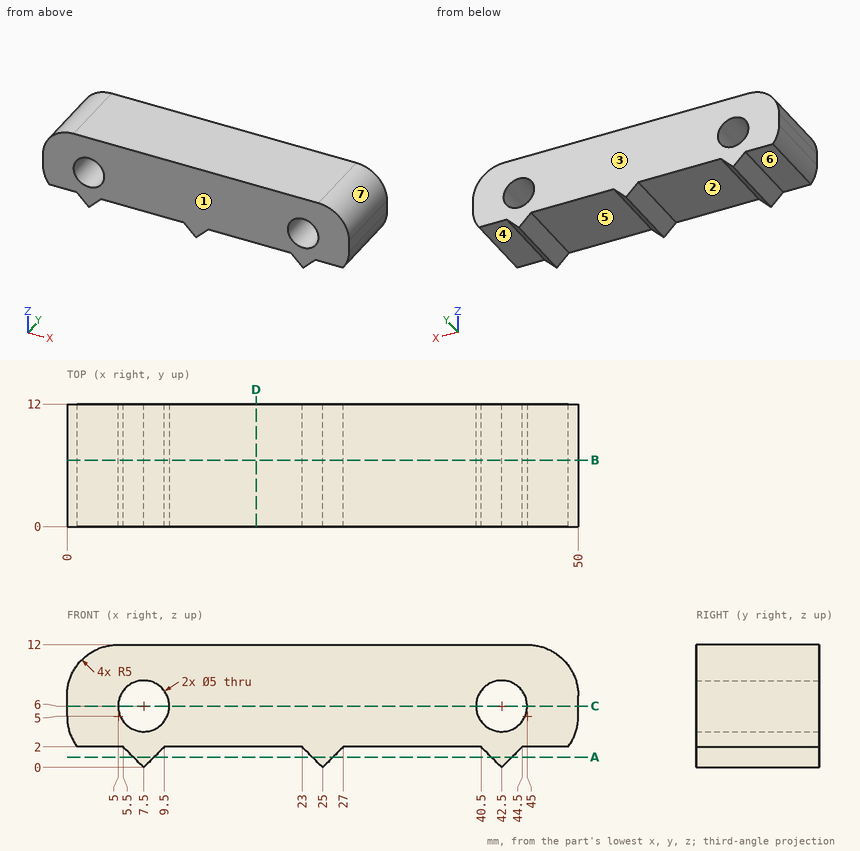
Input: dimensioned drawing with shaded views. Units: mm. Origin: part minimum x, y, z. A direction names the side the tool comes from. Give positions to 0.01 mm unless a question says otherwise; leave off trailing zeros. Write each loop counter-clockwise with the first axis right and the second up, starting at its lowest first coordinate (ties: lowest second). Pieces come first, ordered by that corner, then holes. Notation, with made-up numbers: (-1.5, 3.25) -> (29.5, 3.25) arc R28 ccw to (29.5, 39.25) -> close; hole circle Ø1 at (62, -13). An arc over 180 degrees is marked (long way). Answer as a JSON object with one key per item and string values.
1. Mould query, pull axis Y, two halves, no side actions, for the marked faces 1, 2 and 3. Classes: pulls with the +Y half, pulls with the -Y half, needs draft (parallel to the pull), parting line crosses it, or undercut.
Ans:
{"face 1": "pulls with the -Y half", "face 2": "needs draft", "face 3": "pulls with the +Y half"}
2. Cut plane A-A on z = 1. Output: boundary loops of the cut face in (x, y), and give its area (3 significant figures).
Ans:
{"outline": "(6.5, 0) -> (8.5, 0) -> (8.5, 12) -> (6.5, 12) -> close; (24, 0) -> (26, 0) -> (26, 12) -> (24, 12) -> close; (41.5, 0) -> (43.5, 0) -> (43.5, 12) -> (41.5, 12) -> close", "area": "72.0 mm^2"}
3. Access query for the marked faces 4, 5, 6 and 7. Directions: +Z, -Z, +X, -X, +Y, -Y. A direction counts if a zero-diameter tool reaches every point of the face in a straight line with its end or side. Return the directions, or none.
Ans:
{"face 4": "-Z, +X, +Y, -Y", "face 5": "-Z, +Y, -Y", "face 6": "-Z, -X, +Y, -Y", "face 7": "+Z, +X, +Y, -Y"}
4. Cut plane C-C on z = 6. Output: boundary loops of the cut face in (x, y).
Ans:
{"outline": "(0, 0) -> (5, 0) -> (5, 12) -> (0, 12) -> close; (10, 0) -> (40, 0) -> (40, 12) -> (10, 12) -> close; (45, 0) -> (50, 0) -> (50, 12) -> (45, 12) -> close"}
5. Contact query for flat-ended pins moving along their axis: pin 1 (6 mm diameter, centred on x = 31, y = 5, fed in from -Z); pin 2 (3.5 mm diameter, centred on x = 45.5, y = 7, fed in from -Z); pin 3 (3.5 mm diameter, centred on x = 4, y = 7, fed in from -Z). Output: stop coordinate, or through.
Ans:
{"pin 1": "stops at z = 2", "pin 2": "stops at z = 1.25", "pin 3": "stops at z = 1.75"}
6. Cut plane D-D on x = 18.5. Output: boundary loops of the cut face in (y, z).
Ans:
{"outline": "(0, 2) -> (12, 2) -> (12, 12) -> (0, 12) -> close"}
7. Ray query, probe 1 along X at (y, z) = (6.5, 4.5); probe 2 along X at (y, z) = (6.5, 1.25); probe 3 along Z at (x, y) = (32, 9). Return the intervals inside material, ascending. Write a range as from..to.
Ans:
{"probe 1": "x = 0.03..5.5, 9.5..40.5, 44.5..49.97", "probe 2": "x = 6.25..8.75, 23.75..26.25, 41.25..43.75", "probe 3": "z = 2..12"}
8. Cut plane B-B on y = 6.5. Output: boundary loops of the cut face in (x, z).
Ans:
{"outline": "(0, 5) arc R5 ccw to (1, 2) -> (5.5, 2) -> (7.5, 0) -> (9.5, 2) -> (23, 2) -> (25, 0) -> (27, 2) -> (40.5, 2) -> (42.5, 0) -> (44.5, 2) -> (49, 2) arc R5 ccw to (50, 5) -> (50, 7) arc R5 ccw to (45, 12) -> (5, 12) arc R5 ccw to (0, 7) -> close; hole circle Ø5 at (7.5, 6); hole circle Ø5 at (42.5, 6)"}
